Autodesk Inventor part; units mm, degrees
ref_plane "YZ Plane" through (0, 0, 0) normal (1, 0, 0) x (0, 1, 0)
ref_plane "XZ Plane" through (0, 0, 0) normal (0, 1, 0) x (-1, 0, 0)
ref_plane "XY Plane" through (0, 0, 0) normal (0, 0, 1) x (1, 0, 0)
sketch "草圖1" plane through (0, 0, 0) normal (0, 1, 0) x (-1, 0, 0)
  line L0 (10, 15) -> (-10, 15)
  line L1 (-10, 15) -> (-10, -15)
  line L2 (-5, -20) -> (5, -20)
  line L3 (10, -15) -> (10, 15)
  arc A0 (5, -20) -> (10, -15) centre (5, -15) ccw
  arc A1 (-10, -15) -> (-5, -20) centre (-5, -15) ccw
  circle A2 centre (0, -10) radius 5
  point P0 (0, 0)
  point P1 (10, -20)
  point P2 (0, -20)
  point P3 (10, 0)
  dimension "d0" = 35
  dimension "d1" = 20
  dimension "d2" = 5
  dimension "d3" = 10
  dimension "d4" = 10
extrude "擠出1" add sketch "草圖1" along normal blind 10
sketch "草圖2" plane through (0, 10, 0) normal (0, 1, 0) x (1, 0, 0)
  circle A0 centre (0, 10) radius 5 construction
  line L0 (-10, -15) -> (10, -15) construction
  line L1 (10, -15) -> (10, 15) construction
  arc A1 (10, 15) -> (5, 20) centre (5, 15) ccw construction
  line L2 (5, 20) -> (-5, 20) construction
  arc A2 (-5, 20) -> (-10, 15) centre (-5, 15) ccw construction
  line L3 (-10, 15) -> (-10, -15) construction
  line L4 (10, -15) -> (10, 15)
  line L5 (-10, -15) -> (10, -15)
  line L6 (10, -15) -> (10, -10)
  line L7 (10, -10) -> (-5, -10)
  line L8 (-10, -10.0359) -> (-10, -15)
  line L9 (-10, -15) -> (10, -15)
  line L10 (-10, -15) -> (-6.3427, -15)
  line L11 (-5, -10) -> (-5, 0)
  line L12 (-5, 0) -> (-10, 0)
  line L13 (-10, 0) -> (-10, -15)
  point P0 (0, 0)
  dimension "d7" = 5
  dimension "d8" = 5
  dimension "d9" = 15
extrude "擠出2" add sketch "草圖2" along normal blind 10
sketch "草圖3" plane through (10, 0, 15) normal (1, 0, 0) x (0, 0, -1)
  line L0 (15, 10) -> (5, 10) construction
  line L1 (15, 10) -> (15, 20) construction
  line L2 (5, 20) -> (15, 20) construction
  line L3 (5, 10) -> (5, 20) construction
  line L4 (5, 10) -> (5, 20)
  line L5 (30, 10) -> (15, 10)
  line L6 (5, 20) -> (15, 10)
  line L7 (5, 10) -> (30, 10)
  line L8 (15, 10) -> (5, 10)
  line L9 (5, 10) -> (5, 20)
  point P0 (15, 0)
extrude "擠出3" add sketch "草圖3" against normal blind 5
properties part number "2"
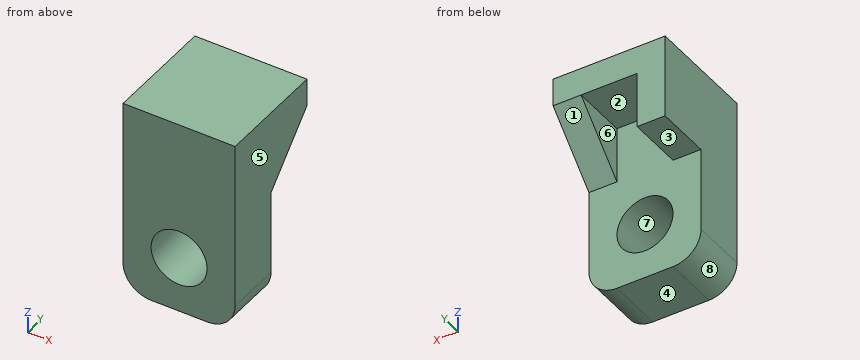
Source: CAD feature listing. Evaluate the final solid. Frame: model axes, mm. Face numbers are marked on the shaded views. A direction names the side the tool comes from. Give positions to 0.01 mm unless a question says otherwise; leave off trailing zeros. Write each loop counter-clockwise with the first axis right and the second up, starting at its lowest first coordinate (ties: lowest second). Pieces come first, ordered by that corner, then holes.
1. Material intervals for line 1 along Z through (x, y) = (0, 4.5); line 2 along Y through (x, z) = (-3, 9.5); line 3 along Z through (x, y) = (4, 9.5), sorted ascending.
2. Access query for the marked faces 1, 2, 3 and 4. Directions: +Z, -Z, +X, -X, +Y, -Y. A direction counts if a zero-diameter tool reaches every point of the face in a straight line with its end or side. Return the directions, or none.
3. Section query A-A (x = -3). Return the cut outline in (y, z), then the cut area to 3 significant figures.
4. Section query D-D (z = 7). Return the cut outline in (x, y), then the cut area to 3 significant figures.
5. Pull-direction query (X, two-part tool) for the marked faces 5, 6, 7 and 8; classes: +X half, -X half, draft (parallel to the pull), parting line (faces both ways), or undercut.
6. First-contact query: pin 1 (4 mm diameter, centred on x = -6.5, y = 13.5, fed in from -Z); pin 2 (8 mm diameter, centred on x = 2.5, z = -15.5, fed in from +Y); pin 3 (2 mm diameter, centred on x = -1, y = 12, fed in from -Z); pin 4 (6 mm diameter, centred on x = 0, z = -10, fed in from -Y). Flat tips, straight axial feed; report the tip coordinate or a pass-through.
7. Section query B-B (y = 2.75). Return the cut outline in (x, z), then the cut area to 3 significant figures.
8. Section query C-C (z = -10). Return the cut outline in (x, y), then the cut area to 3 significant figures.
Output values:
1. line 1: z = -20 to -15, -5 to 15
1. line 2: y = 0 to 10
1. line 3: z = -20 to -13, -7 to 15
2. face 1: -Z, +X, +Y
2. face 2: -Z, +Y
2. face 3: -Z, +X, -X, +Y
2. face 4: -Z, +X, -X, +Y, -Y
3. outline: (0, -20) - (10, -20) - (10, -14) - (0, -14) - close; (0, -6) - (10, -6) - (10, 10) - (20, 10) - (20, 15) - (0, 15) - close
3. area: 320 mm2
4. outline: (-10, 0) - (10, 0) - (10, 17) - (5, 17) - (5, 10) - (-5, 10) - (-5, 20) - (-10, 20) - close
4. area: 285 mm2
5. face 5: +X half
5. face 6: undercut
5. face 7: undercut
5. face 8: -X half
6. pin 1: stops at z = 0
6. pin 2: stops at y = 10
6. pin 3: stops at z = 10
6. pin 4: passes through
7. outline: (-10, -15) arc R5 ccw to (-5, -20) - (5, -20) arc R5 ccw to (10, -15) - (10, 15) - (-10, 15) - close; hole circle Ø10 at (0, -10)
7. area: 611 mm2
8. outline: (-10, 0) - (-5, 0) - (-5, 10) - (-10, 10) - close; (5, 0) - (10, 0) - (10, 10) - (5, 10) - close
8. area: 100 mm2
